```python
from build123d import *

# Parameters (mm, degrees)
SKETCH2_R           = 5
SKETCH2_R_2         = 2.5
BOSS_EXTRUDE1_DEPTH = 6
CHAMFER1_SIZE       = 0.5
SKETCH4_R           = 1
BOSS_EXTRUDE2_DEPTH = 2
CUT_EXTRUDE2_DEPTH  = 0.5
CHAMFER2_SIZE       = 0.5


with BuildPart() as part:
    # Sketch2 → Boss-Extrude1 (new body)
    with BuildSketch(Plane.XY):
        Circle(SKETCH2_R)
        Circle(SKETCH2_R_2, mode=Mode.SUBTRACT)
    extrude(amount=BOSS_EXTRUDE1_DEPTH)

    # Chamfer1
    chamfer1_edges = [part.edges().sort_by_distance(p)[0] for p in [
        (-5, 0, 6),
    ]]
    chamfer(chamfer1_edges, length=CHAMFER1_SIZE)

    # Sketch4 → Boss-Extrude2 (add)
    with BuildSketch(Plane(origin=(0, 4, 0), x_dir=(1, 0, 0), z_dir=(0, 1, 0))):
        with Locations(Location((0, -2.861781198, 0), (0, 0, 90))):
            Circle(SKETCH4_R)
    extrude(amount=BOSS_EXTRUDE2_DEPTH)

    # Sketch5 → Cut-Extrude2 (cut)
    with BuildSketch(Plane(origin=(0, 6, 0), x_dir=(1, 0, 0), z_dir=(0, 1, 0))):
        Polygon((-1.135229539, -3.436253086), (0.891979559, -1.900488617), (1.105020903, -2.181703191), (-0.922188195, -3.71746766), align=None)
    extrude(amount=-CUT_EXTRUDE2_DEPTH, mode=Mode.SUBTRACT)

    # Chamfer2
    chamfer2_edges = [part.edges().sort_by_distance(p)[0] for p in [
        (-5, 0, 0),
    ]]
    chamfer(chamfer2_edges, length=CHAMFER2_SIZE)


solid = part.part
```
Verification items for the finished model (mm, model axes). A direction names the side the tool comes from. Coordinates: 2 decimals unless noted, no trailing zeros. Order: outer loops, then holes, each group sorted by start corner. A loop starts at its lowest first (then second) coordinate and runs counter-clockwise, first axis right, second up. Notation, with made-up numbers: (4.25, 11) -> (23.25, 11) arc R17 cw to (23.25, 31) -> close; hole circle Ø8 at (89.5, 20.5). An arc over 180 degrees is marked (long way). Answer as CSV lines item,"result". Start each with the question number.
1) Set-up check for faces 4 (the face through (2, -2, 6)), 5 (the face through (0.09, 5.75, 2.95)): record each of +Z, -Z, +X, -X, +Y, -Y from which the full face is reachable in a straight line by a thin tool's end or side.
2) Gauge pin test, flat end, axial feed: pin 1 Ø1 at (y, z) = (-3, 0.5) entering from -X. Record the tip position at first contact, or that the pin passes through.
3) Cross-section at D-D, the plane z = 1.25. Record the boundary of the cut face in (x, y).
4) Cross-section at A-A, the plane y = 0. Record the boundary of the cut face in (x, z).
5) Cross-section at B-B, the plane x = 0. Record the boundary of the cut face in (y, z), then the cut area to 3 significant figures.
6) Release check for a two-part mould opening along Z. For faces 1 (the face through (0.383, 5.442, 1.938)), 2 (the face through (-0.15, 5.75, 2.69)), 3 (the face through (-0.4, 6, 2.4)) record: released by +Z, released by -Z, zero draft, split by the parting line, or undercut.
7) Material ranges on L1, parallel to Y at x = 0, z = 1.3; L2, parallel to Y at x = 0, z = 3.4; L3, parallel to X at y = 2, z = 0.6, recorded low to high. Write a range as [from, to].
8) Cross-section at C-C, the plane z = 2.55. Record the boundary of the cut face in (x, y), then the cut area to 3 significant figures.
Conclusion:
1,face 4,"+Z, +X, -X, +Y, -Y"
1,face 5,"+Y"
2,pin 1,"stops at x = -4.33"
3,outline,"circle Ø10 at (0, 0); hole circle Ø5 at (0, 0)"
4,outline,"(-5, 0.5) -> (-4.5, 0) -> (-2.5, 0) -> (-2.5, 6) -> (-4.5, 6) -> (-5, 5.5) -> close; (2.5, 0) -> (4.5, 0) -> (5, 0.5) -> (5, 5.5) -> (4.5, 6) -> (2.5, 6) -> close"
5,outline,"(-5, 0.5) -> (-4.5, 0) -> (-2.5, 0) -> (-2.5, 6) -> (-4.5, 6) -> (-5, 5.5) -> close; (2.5, 0) -> (4.5, 0) -> (5, 0.5) -> (5, 1.86) -> (6, 1.86) -> (6, 2.58) -> (5.5, 2.58) -> (5.5, 3.02) -> (6, 3.02) -> (6, 3.86) -> (5, 3.86) -> (5, 5.5) -> (4.5, 6) -> (2.5, 6) -> close"
5,area,"31.3 mm²"
6,face 1,"split by the parting line"
6,face 2,"undercut"
6,face 3,"zero draft"
7,L1,"y = [-5, -2.5], [2.5, 5]"
7,L2,"y = [-5, -2.5], [2.5, 6]"
7,L3,"x = [-4.58, -1.5], [1.5, 4.58]"
8,outline,"(-0.95, 4.91) arc R5 ccw (long way) to (0.95, 4.91) -> (0.95, 6) -> (0.62, 6) -> (0.62, 5.5) -> (0.03, 5.5) -> (0.03, 6) -> (-0.95, 6) -> close; hole circle Ø5 at (0, 0)"
8,area,"60.6 mm²"
